from build123d import *

# Parameters (mm, degrees)
EXTRUDE_1_DEPTH          = 4
SKETCH_2_W               = 2
SKETCH_2_H               = 15
SKETCH_2_W_2             = 10
SKETCH_2_H_2             = 2
EXTRUDE_2_DEPTH          = 10
SKETCH_3_W               = 20
SKETCH_3_H               = 5
EXTRUDE_3_DEPTH          = 30
SKETCH_4_R               = 1.3
CUT_EXTRUDE_1_DEPTH      = 2
SKETCH_5_R               = 1.3
CUT_EXTRUDE_2_DEPTH      = 59.72818744
CUT_EXTRUDE_3_DEPTH      = 3
SKETCH_7_R               = 1.3
SKETCH_7_R_2             = 2.3
CUT_EXTRUDE_5_DEPTH      = 45.511234537
CUT_EXTRUDE_6_DEPTH      = 2
CUT_EXTRUDE_6_DEPTH_BACK = 2
FILLET_1_R               = 10
FILLET_2_DEPTH           = 4
FILLET_START             = -23.5
FILLET_2_2_DEPTH         = 2
FILLET_START_2           = -24
FILLET_2_3_DEPTH         = 48
FILLET_2_4_DEPTH         = 2
FILLET_3_R               = 5


with BuildPart() as part:
    # 草图1 → 凸台-拉伸1 (new body)
    with BuildSketch(Plane(origin=(0, 0, 0), x_dir=(1, 0, 0), z_dir=(0, 1, 0))):
        Polygon((-21, 23.5), (-21, 4.5), (-23, 4.5), (-23, -10.5), (-21, -10.5), (-21, -18.5), (-11, -18.5), (-10, -18.5), (-10, -23.5), (10, -23.5), (10, -18.5), (11, -18.5), (21, -18.5), (21, -10.5), (23, -10.5), (23, 4.5), (21, 4.5), (21, 23.5), align=None)
    extrude(amount=EXTRUDE_1_DEPTH)

    # 草图2 → 凸台-拉伸2 (add)
    with BuildSketch(Plane(origin=(0, 4, 0), x_dir=(1, 0, 0), z_dir=(0, 1, 0))):
        with Locations((-22, -3)):
            Rectangle(SKETCH_2_W, SKETCH_2_H)
        with Locations((-16, 22.5)):
            Rectangle(SKETCH_2_W_2, SKETCH_2_H_2)
        with Locations((16, 22.5)):
            Rectangle(SKETCH_2_W_2, SKETCH_2_H_2)
        with Locations((22, -3)):
            Rectangle(SKETCH_2_W, SKETCH_2_H)
    extrude(amount=EXTRUDE_2_DEPTH)

    # 草图3 → 凸台-拉伸3 (add)
    with BuildSketch(Plane(origin=(0, 4, 0), x_dir=(1, 0, 0), z_dir=(0, 1, 0))):
        with Locations((0, -21)):
            Rectangle(SKETCH_3_W, SKETCH_3_H)
    extrude(amount=EXTRUDE_3_DEPTH)

    # 草图4 → 切除-拉伸1 (cut)
    with BuildSketch(Plane(origin=(0, 0, -23.5), x_dir=(-1, 0, 0), z_dir=(0, 0, -1))):
        with Locations((-16, 9.5)):
            Circle(SKETCH_4_R)
        with Locations((16, 9.5)):
            Circle(SKETCH_4_R)
    extrude(amount=-CUT_EXTRUDE_1_DEPTH, mode=Mode.SUBTRACT)

    # 草图5 → 切除-拉伸2 (cut, through all)
    with BuildSketch(Plane(origin=(0, 0, 18.5), x_dir=(-1, 0, 0), z_dir=(0, 0, -1))):
        with Locations((0, 25)):
            Circle(SKETCH_5_R)
    extrude(amount=-CUT_EXTRUDE_2_DEPTH, mode=Mode.SUBTRACT)

    # 草图6 → 切除-拉伸3 (cut)
    with BuildSketch(Plane(origin=(0, 0, 18.5), x_dir=(-1, 0, 0), z_dir=(0, 0, -1))):
        Polygon((2.886751346, 25), (1.443375673, 27.5), (-1.443375673, 27.5), (-2.886751346, 25), (-1.443375673, 22.5), (1.443375673, 22.5), align=None)
    extrude(amount=-CUT_EXTRUDE_3_DEPTH, mode=Mode.SUBTRACT)

    # 草图7 → 切除-拉伸5 (cut, through all)
    with BuildSketch(Plane(origin=(0, 4, 0), x_dir=(1, 0, 0), z_dir=(0, 1, 0))):
        with Locations(Location((0, 20.5, 0), (0, 0, 270))):
            Circle(SKETCH_7_R)
        with Locations(Location((-7, 2, 0), (0, 0, 270))):
            Circle(SKETCH_7_R)
        with Locations(Location((7, 2, 0), (0, 0, 270))):
            Circle(SKETCH_7_R)
        with Locations(Location((0, -16.5, 0), (0, 0, 270))):
            Circle(SKETCH_7_R)
        with Locations(Location((-18.5, 2, 0), (0, 0, 270))):
            Circle(SKETCH_7_R_2)
        with Locations(Location((9.5, 17.5, 0), (0, 0, 270))):
            Circle(SKETCH_7_R_2)
        with Locations(Location((9.5, -13.5, 0), (0, 0, 270))):
            Circle(SKETCH_7_R_2)
    extrude(amount=-CUT_EXTRUDE_5_DEPTH, mode=Mode.SUBTRACT)

    # 草图8 → 切除-拉伸6 (cut, two sides: drawn at the far end of the back side and taken through both)
    with BuildSketch(Plane(origin=(0, 4, 0), x_dir=(1, 0, 0), z_dir=(0, 1, 0)).offset(-CUT_EXTRUDE_6_DEPTH_BACK)):
        Polygon((9.886751346, 2), (8.443375673, 4.5), (5.556624327, 4.5), (4.113248654, 2), (5.556624327, -0.5), (8.443375673, -0.5), align=None)
        Polygon((-4.113248654, 2), (-5.556624327, 4.5), (-8.443375673, 4.5), (-9.886751346, 2), (-8.443375673, -0.5), (-5.556624327, -0.5), align=None)
        Polygon((2.886751346, 20.5), (1.443375673, 23), (-1.443375673, 23), (-2.886751346, 20.5), (-1.443375673, 18), (1.443375673, 18), align=None)
        Polygon((2.886751346, -16.5), (1.443375673, -14), (-1.443375673, -14), (-2.886751346, -16.5), (-1.443375673, -19), (1.443375673, -19), align=None)
    extrude(amount=CUT_EXTRUDE_6_DEPTH + CUT_EXTRUDE_6_DEPTH_BACK, mode=Mode.SUBTRACT)

    # 圆角1
    fillet_1_edges = [part.edges().sort_by_distance(p)[0] for p in [
        (-10, 34, 21),
        (10, 34, 21),
    ]]
    fillet(fillet_1_edges, radius=FILLET_1_R - 0.0001)  # a hair under: the kernel refuses the full size

    # 圆角2: read off the stored shape, not the designer's step
    # 圆角2 outline → 圆角2 (add)
    with BuildSketch(Plane(origin=(0, 0, 0), x_dir=(1, 0, 0), z_dir=(0, 1, 0))):
        with BuildLine():
            Line((-21, 4.5), (-21, 8.5))
            ThreePointArc((-21, 8.5), (-21.527864045, 6.263932023), (-23, 4.5))
            Line((-23, 4.5), (-21, 4.5))
        make_face()
        with BuildLine():
            ThreePointArc((21, -14.5), (21.527864045, -12.263932023), (23, -10.5))
            Line((23, -10.5), (21, -10.5))
            Line((21, -10.5), (21, -14.5))
        make_face()
        with BuildLine():
            Line((21, 4.5), (23, 4.5))
            ThreePointArc((23, 4.5), (21.527864045, 6.263932023), (21, 8.5))
            Line((21, 8.5), (21, 4.5))
        make_face()
        with BuildLine():
            Line((-21, -10.5), (-23, -10.5))
            ThreePointArc((-23, -10.5), (-21.527864045, -12.263932023), (-21, -14.5))
            Line((-21, -14.5), (-21, -10.5))
        make_face()
    extrude(amount=FILLET_2_DEPTH)

    # Fillet 2 2 outline → Fillet 2 2 (add)
    with BuildSketch(Plane.XY.offset(FILLET_START)):
        with BuildLine():
            Line((11, 4), (11, 9))
            ThreePointArc((11, 9), (9.535533906, 5.464466094), (6, 4))
            Line((6, 4), (11, 4))
        make_face()
        with BuildLine():
            Line((-11, 4), (-6, 4))
            ThreePointArc((-6, 4), (-9.535533906, 5.464466094), (-11, 9))
            Line((-11, 9), (-11, 4))
        make_face()
    extrude(amount=FILLET_2_2_DEPTH)

    # Fillet 2 3 outline → Fillet 2 3 (cut)
    with BuildSketch(Plane.YZ.offset(FILLET_START_2)):
        with BuildLine():
            Line((14, 10.5), (9, 10.5))
            ThreePointArc((9, 10.5), (12.535533906, 9.035533906), (14, 5.5))
            Line((14, 5.5), (14, 10.5))
        make_face()
        with BuildLine():
            Line((14, -4.5), (14, 0.5))
            ThreePointArc((14, 0.5), (12.535533906, -3.035533906), (9, -4.5))
            Line((9, -4.5), (14, -4.5))
        make_face()
    extrude(amount=FILLET_2_3_DEPTH, mode=Mode.SUBTRACT)

    # Fillet 2 4 outline → Fillet 2 4 (cut)
    with BuildSketch(Plane.XY.offset(FILLET_START)):
        with BuildLine():
            ThreePointArc((16, 14), (19.535533906, 12.535533906), (21, 9))
            Line((21, 9), (21, 14))
            Line((21, 14), (16, 14))
        make_face()
        with BuildLine():
            ThreePointArc((11, 9), (12.464466094, 12.535533906), (16, 14))
            Line((16, 14), (11, 14))
            Line((11, 14), (11, 9))
        make_face()
        with BuildLine():
            ThreePointArc((-16, 14), (-12.464466094, 12.535533906), (-11, 9))
            Line((-11, 9), (-11, 14))
            Line((-11, 14), (-16, 14))
        make_face()
        with BuildLine():
            Line((-21, 14), (-21, 9))
            ThreePointArc((-21, 9), (-19.535533906, 12.535533906), (-16, 14))
            Line((-16, 14), (-21, 14))
        make_face()
    extrude(amount=FILLET_2_4_DEPTH, mode=Mode.SUBTRACT)

    # 圆角3
    # the kernel refuses this fillet: 5 mm, written as the material it adds along each edge
    with BuildSketch(Plane(origin=(10, 0, 18.5), x_dir=(0, 0, 1), z_dir=(0, 1, 0))) as fillet_3_piece_1:
        with BuildLine():
            CenterArc((FILLET_3_R, FILLET_3_R), FILLET_3_R, 180, 90)
            Line((0, FILLET_3_R), (0, 0))
            Line((0, 0), (FILLET_3_R, 0))
        make_face()
    extrude(amount=4)
    with BuildSketch(Plane(origin=(-10, 0, 18.5), x_dir=(0, 0, 1), z_dir=(0, 1, 0))) as fillet_3_piece_2:
        with BuildLine():
            CenterArc((FILLET_3_R, -FILLET_3_R), FILLET_3_R, 90, 90)
            Line((0, -FILLET_3_R), (0, 0))
            Line((0, 0), (FILLET_3_R, 0))
        make_face()
    extrude(amount=4)


solid = part.part
CAD build for the part. Positions are in the model's coordinates, mm. A direction names the side the tool comes from. Coordinates: 2 decimals unless noted, no trailing zeros. Loops run counter-clockwise (first coordinate to the right, second up) from the corner with the lowest first, then second, coordinate; pieces in that order, holes last. Notation, with made-up numbers: (69, -14) -> (78, -14) arc R25 ccw to (78, 24) -> close; hole circle Ø4 at (55.5, 26.5). An arc over 180 degrees is marked (long way). One line per item, written item: value.
1. Slice it at A-A on y = 11.5. Write the cut outline in (x, z), and give its area (3 significant figures).
Answers:
outline: (-23, -3.83) -> (-21, -3.83) -> (-21, 9.83) -> (-23, 9.83) -> close; (-20.33, -23.5) -> (-11.67, -23.5) -> (-11.67, -21.5) -> (-20.33, -21.5) -> close; (-10, 18.5) -> (10, 18.5) -> (10, 23.5) -> (-10, 23.5) -> close; (11.67, -23.5) -> (20.33, -23.5) -> (20.33, -21.5) -> (11.67, -21.5) -> close; (21, -3.83) -> (23, -3.83) -> (23, 9.83) -> (21, 9.83) -> close
area: 189 mm^2
2. Flat gauge pins, fed straight in: P1, Ø0.6, axis at x = 21.5, z = 4, coming from the +Y side; P2, Ø2.5, axis at x = 1, z = 15.5, coming from the +Y side; P3, Ø10, axis at y = 2.5, z = -18, coming from the +X side. Where does each tip first touch, or does it go through?
Answers:
P1: stops at y = 14
P2: stops at y = 4
P3: stops at x = 21
3. Slice it at D-D on y = 15. Write the cut outline in (x, z), and give its area (3 significant figures).
Answers:
outline: (-10, 18.5) -> (10, 18.5) -> (10, 23.5) -> (-10, 23.5) -> close
area: 100 mm^2
4. Slice it at C-C on x = -18.5. Write the cut outline in (y, z).
Answers:
outline: (0, -23.5) -> (13.33, -23.5) -> (13.33, -21.5) -> (4, -21.5) -> (4, -4.3) -> (0, -4.3) -> close; (0, 0.3) -> (4, 0.3) -> (4, 18.5) -> (0, 18.5) -> close
5. Slice it at B-B on z = -17. Write the cut outline in (x, y) (3 decimals), and give its area (3 significant figures).
Answers:
outline: (-21, 0) -> (7.255, 0) -> (7.255, 4) -> (-21, 4) -> close; (11.745, 0) -> (21, 0) -> (21, 4) -> (11.745, 4) -> close
area: 150 mm^2
6. Drill centre lines: line 1 (X direction, y = 2.65, z = -17.5); line 2 (Y direction, x = 0, z = 22.3); line 3 (X direction, y = 1.5, z = -2). Where is each one in solid material? Low to high. Write a range as [from, to].
Answers:
line 1: x = [-21, 7.2], [11.8, 21]
line 2: y = [0, 23.7], [26.3, 34]
line 3: x = [-23, -20.8], [-16.2, -8.3], [-5.7, 5.7], [8.3, 23]
7. Which spindle directions (+Z, -Z, +X, -X, +Y, -Y) get a long thin tool onto all of the face, cutting with end or side? Do faces 1 (the face through (-7, 3, -4.5)), 2 (the face through (21, 2, 17)), 3 (the face through (21, 2, -16)), 4 (the face through (-11.43, 1.97, 20)), 5 (the face through (-8.27, 1.01, -2.28)). Say none if no direction does.
Answers:
face 1: +Y
face 2: +Z, +X, +Y, -Y
face 3: -Z, +X, +Y, -Y
face 4: +Z, -X, +Y, -Y
face 5: +Y, -Y
8. Pull direction Z, two halves, no side cores. Call faces 6 (the face through (-22, 6, -4.5)), 7 (the face through (10.191, 2.028, -15.306)), 8 (the face through (21, 9, 3)), 9 (the face through (0, 3, -18)): pulls with the +Z half, pulls with the -Z half, needs draft (parallel to the pull), parting line crosses it, or undercut.
Answers:
face 6: pulls with the -Z half
face 7: undercut
face 8: needs draft
face 9: undercut
